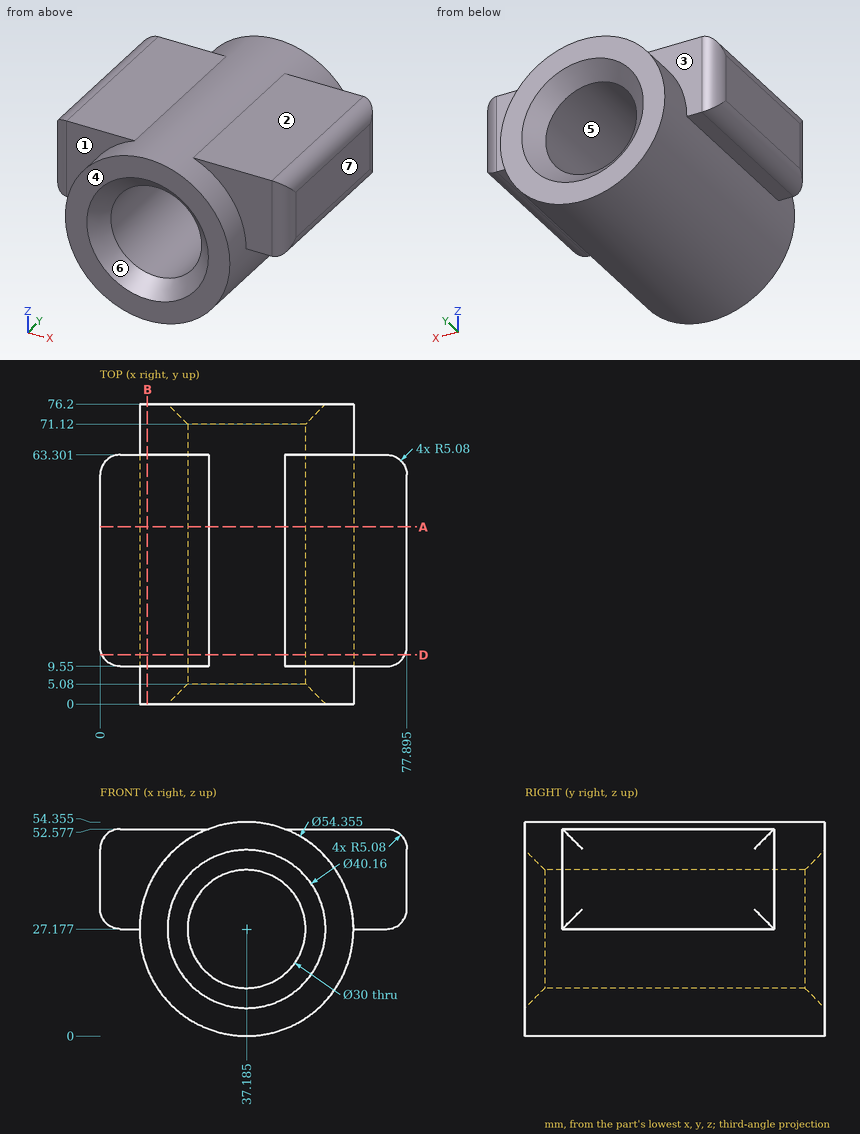
Geometry: see drawing. Coordinates: mm, zero at the bounding-box minimum. A direction names the side the tool comes from. Round coordinates to 2 decimals unless told otherwise and drop trailing zeros. Write each loop counter-clockwise with the first axis right and the second up, starting at its lowest first coordinate (ties: lowest second). Pieces come first, ordered by that corner, then holes.
Item 1: Material intervals for L1, parallel to Y at x = 8.5, z = 31; L2, parallel to X at y = 4, z = 15.5 (1 decimal); L3, parallel to Z at x = 39, y = 23.5 (1 decimal), sorted ascending.
Item 2: Section query D-D (y = 12.5). Return loops of the section in (x, z) (1 decimal).
Item 3: Section query B-B (x = 12). Return loops of the section in (y, z).
Item 4: Pin query (flat end, axial travel): P1, Ø18, axis at x = 20.5, y = 36, coming from the +Z side (1 decimal); P2, Ø7, axis at x = 70.5, y = 25, coming from the -Z side; P3, Ø2, axis at x = 39, y = 55, coming from the -Z side. Return the tip coordinate at first contact, or that it passes through.
Item 5: Mould query, pull axis X, two halves, no side actions, for the marked faces 4, 5, 6 and 7. Classes: +X half, -X half, draft (parallel to the pull), parting line (faces both ways), or undercut.
Item 6: Section query A-A (y = 45). Return loops of the section in (x, z) (1 decimal), plus the area to 3 significant figures.
Item 7: Set-up query: the marked faces 1, 2 and 3. Return all of +Z, -Z, +X, -X, +Y, -Y with unobstructed straight access to the full face (end or side cutting, diameter ignored); none if empty.
Completed:
1. L1: y = 9.55 to 63.3
1. L2: x = 12.6 to 26.1, 48.2 to 61.7
1. L3: z = 0.1 to 12.3, 42.1 to 54.3
2. outline: (0.5, 30.1) arc R5.1 ccw to (5.1, 27.2) - (10, 27.2) arc R27.2 ccw to (64.4, 27.2) - (72.8, 27.2) arc R5.1 ccw to (77.4, 30.1) - (77.4, 49.6) arc R5.1 ccw to (72.8, 52.6) - (46.9, 52.6) arc R27.2 ccw to (27.5, 52.6) - (5.1, 52.6) arc R5.1 ccw to (0.5, 49.6) - close; hole circle Ø30 at (37.2, 27.2)
3. outline: (0, 16.96) - (76.2, 16.96) - (76.2, 37.39) - (63.3, 37.39) - (63.3, 52.58) - (9.55, 52.58) - (9.55, 37.39) - (0, 37.39) - close
4. P1: stops at z = 53.2
4. P2: stops at z = 27.18
4. P3: stops at z = 0.01
5. face 4: draft
5. face 5: undercut
5. face 6: undercut
5. face 7: +X half
6. outline: (0, 32.3) arc R5.1 ccw to (5.1, 27.2) - (10, 27.2) arc R27.2 ccw to (64.4, 27.2) - (72.8, 27.2) arc R5.1 ccw to (77.9, 32.3) - (77.9, 47.5) arc R5.1 ccw to (72.8, 52.6) - (46.9, 52.6) arc R27.2 ccw to (27.5, 52.6) - (5.1, 52.6) arc R5.1 ccw to (0, 47.5) - close; hole circle Ø30 at (37.2, 27.2)
6. area: 2,430 mm2
7. face 1: +Z, -X, -Y
7. face 2: +Z, +X, +Y, -Y
7. face 3: +Z, -X, +Y
